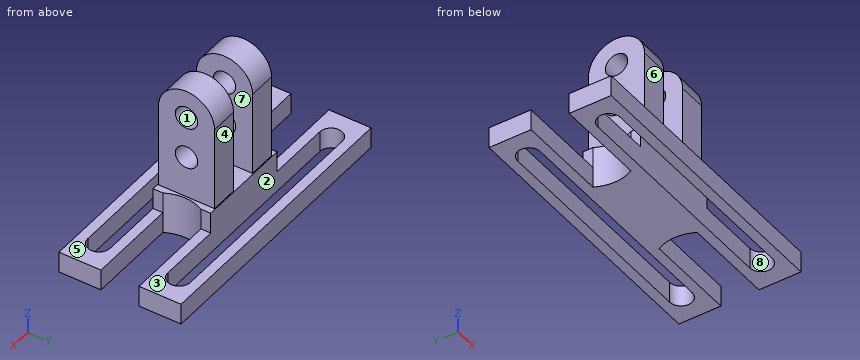
```python
from build123d import *

# Parameters (mm, degrees)
EXTRUDE_1_DEPTH = 3
EXTRUDE_2_DEPTH = 3
EXTRUDE_START   = 2
SKETCH_3_R      = 1.6
EXTRUDE_3_DEPTH = 4


with BuildPart() as part:
    # 草图1 → 凸台-拉伸1 (new body)
    with BuildSketch(Plane.XY):
        with BuildLine():
            Line((20, 8.715), (20, 2.715))
            Line((20, 2.715), (6.971083616, 2.715))
            ThreePointArc((6.971083616, 2.715), (6.285, 0), (6.971083616, -2.715))
            Line((6.971083616, -2.715), (20, -2.715))
            Line((20, -2.715), (20, -8.715))
            Line((20, -8.715), (-20, -8.715))
            Line((-20, -8.715), (-20, -2.715))
            Line((-20, -2.715), (-6.971083616, -2.715))
            ThreePointArc((-6.971083616, -2.715), (-6.285, 0), (-6.971083616, 2.715))
            Line((-6.971083616, 2.715), (-20, 2.715))
            Line((-20, 2.715), (-20, 8.715))
            Line((-20, 8.715), (20, 8.715))
        make_face()
        with BuildLine():
            Line((16, 4.115), (-16, 4.115))
            ThreePointArc((-16, 4.115), (-17.6, 5.715), (-16, 7.315))
            Line((-16, 7.315), (16, 7.315))
            ThreePointArc((16, 7.315), (17.6, 5.715), (16, 4.115))
        make_face(mode=Mode.SUBTRACT)
        with BuildLine():
            Line((16, -7.315), (-16, -7.315))
            ThreePointArc((-16, -7.315), (-17.6, -5.715), (-16, -4.115))
            Line((-16, -4.115), (16, -4.115))
            ThreePointArc((16, -4.115), (17.6, -5.715), (16, -7.315))
        make_face(mode=Mode.SUBTRACT)
    extrude(amount=EXTRUDE_1_DEPTH)

    # 草图2 → 凸台-拉伸2 (add)
    with BuildSketch(Plane.XY.offset(3)):
        with BuildLine():
            Line((-6.971083616, 2.715), (-6.971083616, 4.115))
            Line((-6.971083616, 4.115), (6.971083616, 4.115))
            Line((6.971083616, 4.115), (6.971083616, 2.715))
            ThreePointArc((6.971083616, 2.715), (6.285, 0), (6.971083616, -2.715))
            Line((6.971083616, -2.715), (6.971083616, -4.115))
            Line((6.971083616, -4.115), (-6.971083616, -4.115))
            Line((-6.971083616, -4.115), (-6.971083616, -2.715))
            ThreePointArc((-6.971083616, -2.715), (-6.285, 0), (-6.971083616, 2.715))
        make_face()
    extrude(amount=EXTRUDE_2_DEPTH)

    # 草图3 → 凸台-拉伸3 (add)
    with BuildSketch(Plane(origin=(0, 0, 0), x_dir=(0, 0, -1), z_dir=(1, 0, 0)).offset(EXTRUDE_START)):
        with BuildLine():
            Line((-6, 4), (-18, 4))
            ThreePointArc((-18, 4), (-22, 0), (-18, -4))
            Line((-18, -4), (-6, -4))
            Line((-6, -4), (-6, 4))
        make_face()
        with Locations((-18, 0)):
            Circle(SKETCH_3_R, mode=Mode.SUBTRACT)
        with Locations((-12, 0)):
            Circle(SKETCH_3_R, mode=Mode.SUBTRACT)
    extrude_3 = extrude(amount=EXTRUDE_3_DEPTH)

    # 镜向1: 凸台-拉伸3 across plane
    add(extrude_3.mirror(Plane(origin=(0, 0, 0), x_dir=(0, 0, 1), z_dir=(1, 0, 0))))


solid = part.part
```
Geometry: final body of the model. Coordinates: model frame, mm. Face numbers are marked on the shaded views. A direction names the side the tool comes from. Round coordinates to 2 decimals unless told otherwise and drop trailing zeros. Write each loop counter-clockwise with the first axis right and the second up, starting at its lowest first coordinate (ties: lowest second). Pieces come first, ordered by that corner, then holes. Notation, with made-up numbers: M 78.5,-40 L 132.5,-40 A31 ccw 132.5,-1 Z; hole C -36,-10.75 d3. An arc over 180 degrees is marked long. Answer in a Markdown table with one row per item. Add a question column.
(1) Ray query, L1, parallel to Y at x = 3.15, z = 18; L2, parallel to X at y = 1.75, z = 9.5; L3, parallel to Y at x = 2.5, z = 6.75. Return the intervals inside material, ascending.
(2) Cut plane C-C, the plane z = 7. Return the cut outline in (x, y).
(3) Cut plane A-A, the plane x = 5.5. Return the cut outline in (y, z) (3 decimals).
(4) Cut plane B-B, the plane x = 13.5. Return the cut outline in (y, z) (3 decimals).
(5) Reachability of the marked faces 4, 5, 6, 7 and 8 from +Z, -Z, +X, -X, +Y, -Y: full face, straight path, thin tool, end or side. Return the list, or none.
(6) Draft query along Z for the marked faces 1, 2 and 3. Return one class per face: pulls with the +Z half, pulls with the -Z half, needs draft (parallel to the pull), parting line crosses it, or undercut.
(7) Contact query for flat-ended pins moving along their axis: pin 1 (5 mm diameter, centred on x = 9.5, y = 2.5, fed in from -Z); pin 2 (4 mm diameter, centred on y = 0, z = 12, fed in from +X); pin 3 (5 mm diameter, centred on y = 0, z = 18, fed in from -X); pin 4 (2.5 mm diameter, centred on x = -0.5, y = 0, fed in from +Z). Output: stop coordinate, or through.
(8) Cut plane D-D, the plane y = 0. Return the cut outline in (x, z) (3 decimals).
Established:
| question | item | result |
|---|---|---|
| 1 | L1 | -4 to -1.6, 1.6 to 4 |
| 1 | L2 | -6 to -2, 2 to 6 |
| 1 | L3 | -4 to 4 |
| 2 | outline | M -6,-4 L -2,-4 L -2,4 L -6,4 Z; M 2,-4 L 6,-4 L 6,4 L 2,4 Z |
| 3 | outline | M -8.715,0 L -7.315,0 L -7.315,3 L -8.715,3 Z; M -4.115,0 L 4.115,0 L 4.115,6 L 4,6 L 4,18 A4 ccw -4,18 L -4,6 L -4.115,6 Z; M 7.315,0 L 8.715,0 L 8.715,3 L 7.315,3 Z; hole C 0,12 d3.2; hole C 0,18 d3.2 |
| 4 | outline | M -8.715,0 L -7.315,0 L -7.315,3 L -8.715,3 Z; M -4.115,0 L -2.715,0 L -2.715,3 L -4.115,3 Z; M 2.715,0 L 4.115,0 L 4.115,3 L 2.715,3 Z; M 7.315,0 L 8.715,0 L 8.715,3 L 7.315,3 Z |
| 5 | face 4 | +Z, +X, -X, +Y |
| 5 | face 5 | +Z, -Y |
| 5 | face 6 | +Z, +X, -X, -Y |
| 5 | face 7 | +Z, +Y, -Y |
| 5 | face 8 | +Z, -Z |
| 6 | face 1 | undercut |
| 6 | face 2 | needs draft |
| 6 | face 3 | pulls with the +Z half |
| 7 | pin 1 | z = 0 |
| 7 | pin 2 | x = 6 |
| 7 | pin 3 | x = -6 |
| 7 | pin 4 | z = 6 |
| 8 | outline | M -6.285,0 L 6.285,0 L 6.285,6 L 6,6 L 6,10.4 L 2,10.4 L 2,6 L -2,6 L -2,10.4 L -6,10.4 L -6,6 L -6.285,6 Z; M -6,13.6 L -2,13.6 L -2,16.4 L -6,16.4 Z; M -6,19.6 L -2,19.6 L -2,22 L -6,22 Z; M 2,13.6 L 6,13.6 L 6,16.4 L 2,16.4 Z; M 2,19.6 L 6,19.6 L 6,22 L 2,22 Z |
